from build123d import *

# Parameters (mm, degrees)
F0_R     = 3.81
F1_DEPTH = 25.4
F0_W     = 177.8
F0_H     = 12.7
F0_R_2   = 1.27
F2_DEPTH = 6.35
F3_D     = 3.429
F4_D     = 7.62


with BuildPart() as f1:
    # F0 (on Front) → F1 (new body)
    with BuildSketch(Plane.XZ):
        with Locations((76.2, 0)):
            Circle(F0_R)
    extrude(amount=F1_DEPTH)

    # F0 (on Front) → F2 (join)
    with BuildSketch(Plane.XZ):
        Rectangle(F0_W, F0_H)
        with Locations((-76.2, 0)):
            Circle(F0_R_2, mode=Mode.SUBTRACT)
        with Locations((-25.4, 0)):
            Circle(F0_R_2, mode=Mode.SUBTRACT)
        with Locations((76.2, 0)):
            Circle(F0_R, mode=Mode.SUBTRACT)
        with Locations((-25.4, 0)):
            Circle(F0_R_2)
        with Locations((-76.2, 0)):
            Circle(F0_R_2)
    extrude(amount=F2_DEPTH)

    # F3 (through all)
    with Locations(Plane(origin=(0, 0, 0), x_dir=(1, 0, 0), z_dir=(0, 1, 0))):
        with Locations((-25.4, 0), (-76.2, 0)):
            Hole(F3_D / 2)

    # F4 (through all)
    with Locations(Plane(origin=(0, 0, 0), x_dir=(1, 0, 0), z_dir=(0, 1, 0))):
        with Locations((76.2, 0)):
            Hole(F4_D / 2)


solid = f1.part
The model under review builds one solid part; all positions refer to its coordinate system, in mm. Give positions to 0.01 mm unless a question says otherwise; leave off trailing zeros. Write each loop counter-clockwise with the first axis right and the second up, starting at its lowest first coordinate (ties: lowest second). Pieces come first, ordered by that corner, then holes.
1. Add section D-D, the plane x = 76.2. Write out the cut boundary in (y, z), plus the area to 3 significant figures.
2. Add section C-C, the plane z = 0. Write out the cut boundary in (x, y).
3. Add section B-B, the plane x = -76.2. Write out the cut boundary in (y, z), plus the area to 3 significant figures.
4. Wall thickness on L1, parallel to Z at x = -76.2, y = -4.5; L2, parallel to X at y = -3, z = 1.5; L3, parallel to Z at x = 76.2, y = -1.5: over which ranges is each line inside the solid? List them lowest first.
5. Draft analysis for pull direction X (two halves, no side actions). For faces 1 (the flat face through (-88.9, -3, 0)), 2 (the cylindrical face through (80.006, -3.219, -0.168)), 3 (the flat face through (-1, -6.35, 0)), 4 (the cylindrical face through (-74.487, -3.219, -0.075)), state which applies: +X half, -X half, draft (parallel to the pull), parting line (faces both ways), or undercut.
6. Add section A-A, the plane y = -5. Write out the cut boundary in (x, z), plus the area to 3 significant figures.
Worked answers:
1. outline: (-6.35, -6.35) - (0, -6.35) - (0, -3.81) - (-6.35, -3.81) - close; (-6.35, 3.81) - (0, 3.81) - (0, 6.35) - (-6.35, 6.35) - close
1. area: 32.3 mm2
2. outline: (-88.9, -6.35) - (-77.91, -6.35) - (-77.91, 0) - (-88.9, 0) - close; (-74.49, -6.35) - (-27.11, -6.35) - (-27.11, 0) - (-74.49, 0) - close; (-23.69, -6.35) - (72.39, -6.35) - (72.39, 0) - (-23.69, 0) - close; (80.01, -6.35) - (88.9, -6.35) - (88.9, 0) - (80.01, 0) - close
3. outline: (-6.35, -6.35) - (0, -6.35) - (0, -1.71) - (-6.35, -1.71) - close; (-6.35, 1.71) - (0, 1.71) - (0, 6.35) - (-6.35, 6.35) - close
3. area: 58.9 mm2
4. L1: z = -6.35 to -1.71, 1.71 to 6.35
4. L2: x = -88.9 to -77.03, -75.37 to -26.23, -24.57 to 72.7, 79.7 to 88.9
4. L3: z = -6.35 to -3.81, 3.81 to 6.35
5. face 1: -X half
5. face 2: undercut
5. face 3: draft
5. face 4: undercut
6. outline: (-88.9, -6.35) - (88.9, -6.35) - (88.9, 6.35) - (-88.9, 6.35) - close; hole circle Ø3.43 at (-76.2, 0); hole circle Ø3.43 at (-25.4, 0); hole circle Ø7.62 at (76.2, 0)
6. area: 2,190 mm2
